from build123d import *

# Parameters (mm, degrees)
SKETCH_1_W      = 34
SKETCH_1_H      = 34
SKETCH_1_W_2    = 28
SKETCH_1_H_2    = 28
EXTRUDE_1_DEPTH = 34
EXTRUDE_2_REACH = 33
SKETCH_2_W      = 3
SKETCH_2_H      = 28


with BuildPart() as part:
    # 草图1 → 凸台-拉伸1 (new body)
    with BuildSketch(Plane.XY):
        Rectangle(SKETCH_1_W, SKETCH_1_H)
        Rectangle(SKETCH_1_W_2, SKETCH_1_H_2, mode=Mode.SUBTRACT)
    extrude(amount=EXTRUDE_1_DEPTH)

    # 草图2 → 凸台-拉伸2 (add, up to next)
    with BuildSketch(Plane(origin=(-14, 0, 0), x_dir=(0, 0, -1), z_dir=(1, 0, 0)), mode=Mode.PRIVATE) as extrude_2_sk1:
        with Locations((-1.5, 0)):
            Rectangle(SKETCH_2_W, SKETCH_2_H)
    extrude_2_tool1 = extrude(extrude_2_sk1.sketch, amount=EXTRUDE_2_REACH, mode=Mode.PRIVATE) - part.part
    add(extrude_2_tool1.solids().sort_by_distance((-14, 0, 1.5))[0])


solid = part.part
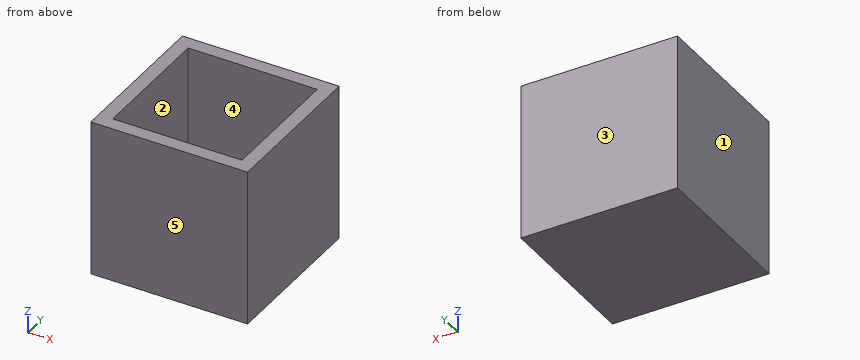
Input: part model. Units: mm. Frame: model coordinates. Face numbers are marked on the shaded views. A direction names the side the tool comes from. Coordinates: 2 decimals unless noted, no trailing zeros. Order: outer loops, then holes, each group sorted by start corner. A loop starts at its lowest first (then second) coordinate and runs counter-clockwise, first axis right, second up. Notation, with made-up numbers: M -19,59 L 5,59 A8 cw 5,65 Z; hole C -17.5,36.25 d4. An arc over 180 degrees is marked long. One line per question, with ' | ' between items.
Item 1: Reachability of the marked faces 4 and 5 from +Z, -Z, +X, -X, +Y, -Y: full face, straight path, thin tool, end or side. Return the list, or none.
Geometry results:
face 4: +Z | face 5: +Z, -Z, +X, -X, -Y
Item 2: Section B-B (y = 10). Output: boundary loops of the cut face in (x, z), then the cut area to 3 significant figures.
Geometry results:
outline: M -17,0 L 17,0 L 17,34 L 14,34 L 14,3 L -14,3 L -14,34 L -17,34 Z | area: 288 mm^2
Item 3: Ray query, line 1 along Y through (x, z) = (-3, 15); line 2 along Z through (x, y) = (-2.5, 13.5). Return the intervals inside material, ascending.
Geometry results:
line 1: y = -17 to -14, 14 to 17 | line 2: z = 0 to 3
Item 4: Section A-A (z = 23.5). Output: boundary loops of the cut face in (x, y), then the cut area to 3 significant figures.
Geometry results:
outline: M -17,-17 L 17,-17 L 17,17 L -17,17 Z; hole M -14,-14 L 14,-14 L 14,14 L -14,14 Z | area: 372 mm^2
Item 5: Draft query along X for the marked faces 1, 2 and 3. Return one class per face: released by +X, released by -X, zero draft, split by the parting line, or undercut.
Geometry results:
face 1: released by -X | face 2: undercut | face 3: zero draft
Item 6: Pin query (flat end, axial travel): pin 1 (10 mm diameter, centred on x = 11.5, y = 13.5, fed in from -Z); pin 2 (6 mm diameter, centred on x = -10, y = -2.5, fed in from +Z). Return the tip coordinate at first contact, or that it passes through.
Geometry results:
pin 1: stops at z = 0 | pin 2: stops at z = 3
